The model under review builds one solid part; all positions refer to its coordinate system, in mm. Face numbers are marked on the shaded views. A direction names the side the tool comes from. Round coordinates to 2 decimals unless told otherwise and drop trailing zeros. Loops run counter-clockwise (first coordinate to the right, second up) from the corner with the lowest first, then second, coordinate; pieces in that order, holes last. Notation, with made-up numbers: (-19, 71.5) -> (-9, 71.5) arc R31 cw to (-9, 108.5) -> close; hole circle Ø7 at (3.25, 8.5). An arc over 180 degrees is marked (long way). Use a Markdown table: item, result. Add a question column.
1) For the marked faces 4 and 5, list the 3-axis set-ups (+Z, -Z, +X, -X, +Y, -Y) from which the entire face can be reached by the end or side of a thin tool; tool diameter is ignored.
2) Consider section B-B on z = 10.5. Give the boundary of the cut face in (x, y).
3) Mouldability with a two-part tool opening along X and no side actions: class the marked faces 1, 2 and 3 as released by +X, released by -X, zero draft, split by the parting line, or undercut.
4) Wall thickness on probe 1 along Z at (x, y) = (11.25, 10); probe 2 along X at (y, z) = (4.5, -18); probe 3 along Y at (x, z) = (-7.5, -27.5): over which ranges is each line inside the solid? List them lowest first.
5) Consider section A-A on z = 20. State how many separate pieces and enclosed holes the cut face has, plus the area to 3 significant figures.
6) Consider section D-D on y = 5.5. Give the boundary of the cut face in (x, z), plus the area to 3 significant figures.
7) Insertion check: pin 1 (0.9 mm diameter, centred on x = 1.5, y = -10, fed in from -Z); pin 2 (5 mm diameter, centred on x = -7.24, y = 4.76, fed in from +Z); pin 3 (6.5 mm diameter, centred on y = -17.51, z = 20, fed in from +X); pin 4 (3 mm diameter, centred on x = 7.5, y = -12.5, fed in from +Z). Each pin has a flat end and moves straight along its axis. Give the tip position at first contact, or say it passes through.
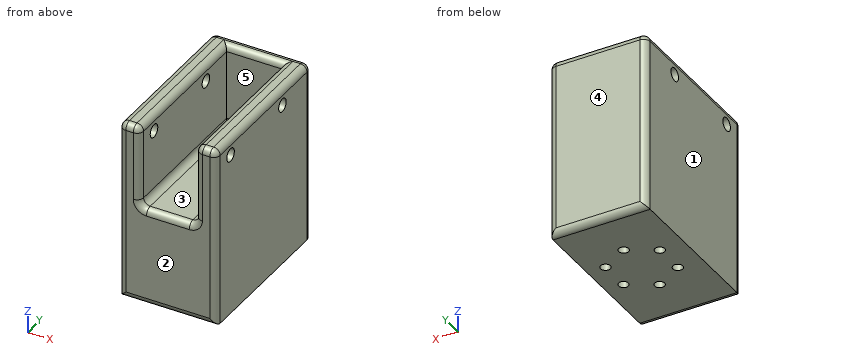
from build123d import *

# Parameters (mm, degrees)
F1_DEPTH  = 25
F2_DEPTH  = 5
F3_DEPTH  = 25
F4_R      = 2
F5_DEPTH  = 29.5357977842
F6_R      = 2
F7_DEPTH  = 29.5357977842
F8_R      = 1.99999
F9_R      = 1.5
F10_DEPTH = 15


# Not quite as in the source:
# - a fillet or chamfer is up to 0.001 mm smaller than in the source, because OpenCascade refuses the exact size
# - a feature names something its author has since deleted; it is built from what else it names


with BuildPart() as f1:
    # F0 (on Top) → F1 (new body)
    with BuildSketch(Plane.XY):
        Polygon((-8.5, -23.510635891), (-8.5, 0), (-8.5, 21), (8.5, 21), (8.5, 0), (8.5, -23.510635891), (8.5, -25), (14.7673988921, -25), (14.7673988921, -20.1723555878), (14.7673988921, -13.510635891), (14.7673988921, 25), (-14.7673988921, 25), (-14.7673988921, -20.1723555878), (-14.7673988921, -25), (-8.5, -25), align=None)
    extrude(amount=F1_DEPTH)

    # F0 (on Top) → F2 (join)
    with BuildSketch(Plane.XY):
        Polygon((-8.5, 21), (-8.5, 0), (-8.5, -23.510635891), (-8.5, -25), (8.5, -25), (8.5, -23.510635891), (8.5, 0), (8.5, 21), align=None)
        Polygon((-8.5, -23.510635891), (-8.5, 0), (-8.5, 21), (8.5, 21), (8.5, 0), (8.5, -23.510635891), (8.5, -25), (14.7673988921, -25), (14.7673988921, -20.1723555878), (14.7673988921, -13.510635891), (14.7673988921, 25), (-14.7673988921, 25), (-14.7673988921, -20.1723555878), (-14.7673988921, -25), (-8.5, -25), align=None)
    extrude(amount=-F2_DEPTH)

    # F3 (add): a face of the model
    f3_faces = [f1.faces().sort_by_distance(p)[0] for p in [
        (0, 0, -5),
    ]]
    extrude(f3_faces, amount=F3_DEPTH)

    # F4 (on face) → F5 (cut, through all)
    with BuildSketch(Plane.YZ.offset(14.7673988921)):
        with Locations((10, 20)):
            Circle(F4_R)
    extrude(amount=-F5_DEPTH, mode=Mode.SUBTRACT)

    # F6 (on face) → F7 (cut, through all)
    with BuildSketch(Plane.YZ.offset(14.7673988921)):
        with Locations((-17.510635891, 20)):
            Circle(F6_R)
    extrude(amount=-F7_DEPTH, mode=Mode.SUBTRACT)

    # F8 (radius 2 in the source; OpenCascade refuses exactly that, so slightly less here)
    f8_edges = [f1.edges().sort_by_distance(p)[0] for p in [
        (-11.633699, -25, 25),
        (-8.5, -2, 25),
        (0, 21, 25),
        (8.5, -2, 25),
        (11.633699, -25, 25),
        (14.767399, 0, 25),
        (0, 25, 25),
        (-14.767399, 0, 25),
        (-14.767399, 25, -2.5),
        (0, 25, -30),
        (14.767399, 25, -2.5),
        (-14.767399, -25, -2.5),
        (-8.5, -25, 12.5),
        (0, -25, 0),
        (8.5, -25, 12.5),
        (14.767399, -25, -2.5),
        (0, -25, -30),
        (-8.5, -2, 0),
        (0, 21, 0),
        (8.5, -2, 0),
    ]]
    fillet(f8_edges, radius=F8_R)

    # F9 (on face) → F10 (cut)
    with BuildSketch(Plane(origin=(0, 0, -30), x_dir=(1, 0, 0), z_dir=(0, 0, -1))):
        with Locations((9.2546826823, -4.7625)):
            Circle(F9_R)
        with Locations((1.0057907112, -9.525)):
            Circle(F9_R)
        with Locations((-7.2431012598, -4.7625)):
            Circle(F9_R)
        with Locations((-7.2431012598, 4.7625)):
            Circle(F9_R)
        with Locations((1.0057907112, 9.525)):
            Circle(F9_R)
        with Locations((9.2546826823, 4.7625)):
            Circle(F9_R)
    extrude(amount=-F10_DEPTH, mode=Mode.SUBTRACT)


solid = f1.part
Result set:
| question | item | result |
|---|---|---|
| 1 | face 4 | +Z, -Z, +X, -X, +Y |
| 1 | face 5 | +Z, -Y |
| 2 | outline | (-14.77, -23) arc R2 ccw to (-12.77, -25) -> (-10.5, -25) arc R2 ccw to (-8.5, -23) -> (-8.5, 21) -> (8.5, 21) -> (8.5, -23) arc R2 ccw to (10.5, -25) -> (12.77, -25) arc R2 ccw to (14.77, -23) -> (14.77, 23) arc R2 ccw to (12.77, 25) -> (-12.77, 25) arc R2 ccw to (-14.77, 23) -> close |
| 3 | face 1 | released by -X |
| 3 | face 2 | zero draft |
| 3 | face 3 | undercut |
| 4 | probe 1 | -30 to 18, 22 to 25 |
| 4 | probe 2 | -14.77 to -8.72, -5.77 to 7.78, 10.73 to 14.77 |
| 4 | probe 3 | -25 to -6.24, -3.28 to 3.28, 6.24 to 25 |
| 5 | separate pieces | 5 |
| 5 | enclosed holes | 0 |
| 5 | area | 589 mm2 |
| 6 | outline | (-14.77, -30) -> (-8.55, -30) -> (-8.55, -15) -> (-5.94, -15) -> (-5.94, -30) -> (7.95, -30) -> (7.95, -15) -> (10.56, -15) -> (10.56, -30) -> (14.77, -30) -> (14.77, 23) arc R2 ccw to (12.77, 25) -> (10.5, 25) arc R2 ccw to (8.5, 23) -> (8.5, 2) arc R2 cw to (6.5, 0) -> (-6.5, 0) arc R2 cw to (-8.5, 2) -> (-8.5, 23) arc R2 ccw to (-10.5, 25) -> (-12.77, 25) arc R2 ccw to (-14.77, 23) -> close |
| 6 | area | 1,120 mm2 |
| 7 | pin 1 | z = -15 |
| 7 | pin 2 | z = 24.85 |
| 7 | pin 3 | x = 14.77 |
| 7 | pin 4 | z = 24.32 |
